Read the model definition and answer for the solid it produces. Units are mm, in the model's axes. Face numbers are marked on the shaded views. A direction names the side the tool comes from. Coordinates: 2 decimals unless noted, no trailing zeros. Loops run counter-clockwise (first coordinate to the right, second up) from the corner with the lowest first, then second, coordinate; pieces in that order, holes last. Notation, with made-up numbers: (-40, -24.75) -> (-9, -24.75) arc R20 cw to (-9, -18.75) -> close; hole circle Ø3 at (-19.5, 78). An arc over 180 degrees is marked (long way). Answer as a JSON object with one key per item and string values. Group by question number.
1) Section A-A, the plane y = 0 is taken. Give the vertices of the cut face in (x, z), plus the area to 3 significant figures.
2) Section D-D, the plane x = -38.5 is taken. Give the vertices of the cut face in (y, z).
3) Flat-ended cylindrical pins translate along their axes: P1, Ø4, axis at x = -9.5, z = 15.5, coming from the +Y side; P2, Ø4, axis at x = 33.64, y = 46.31, coming from the +Z side; P3, Ø6.5, axis at x = 54.44, y = -17.69, coming from the +Z side; P4, Ø2, axis at y = -8.5, z = 6.5, coming from the +X side. Find the tip coordinate at first contact, or state that the pin passes through.
4) Determine the mould class of the marked faces 4, 5 and 6 for opening direction X: released by +X, released by -X, zero draft, split by the parting line, or undercut.
5) Consider probe 1 along Y at (x, z) = (-35.5, 4.75); probe 2 along Y at (x, z) = (-0.5, 4.75); probe 3 along Z at (x, y) = (-25, 16). Determine where each line is inside the solid, lowest interval first. Write a range as [from, to].
6) Section B-B, the plane x = 0 is taken. Count the separate pieces of the cut face and the enclosed holes in it, plus the area to 4 significant figures.
7) Section C-C, the plane z = 9.25 is taken. Give the vertices of the cut face in (x, y), plus the area to 3 significant figures.
8) Which of the six approach directions +Z, -Z, +X, -X, +Y, -Y give full straight-line access (tool end or side, diameter ignored) to the marked faces 1, 2 and 3?
from build123d import *

# Parameters (mm, degrees)
SKETCH1_R           = 63.5
BOSS_EXTRUDE1_DEPTH = 5
SKETCH2_R           = 51
BOSS_EXTRUDE2_DEPTH = 13
SKETCH3_R           = 36
CUT_EXTRUDE1_DEPTH  = 19
CUT_EXTRUDE3_START  = -2.5
SKETCH4_R           = 37.5
SKETCH4_R_2         = 36
CUT_EXTRUDE3_DEPTH  = 2
SKETCH6_R           = 36
SKETCH6_R_2         = 34
BOSS_EXTRUDE6_DEPTH = 2
SKETCH9_R           = 2.5
CUT_EXTRUDE9_DEPTH  = 6
SKETCH10_R          = 2.5
CUT_EXTRUDE10_DEPTH = 19
CUT_EXTRUDE11_DEPTH = 19
FILLET1_R           = 3
FILLET2_R           = 3
FILLET3_R           = 3


with BuildPart() as part:
    # Sketch1 → Boss-Extrude1 (new body)
    with BuildSketch(Plane.XY):
        Circle(SKETCH1_R)
    extrude(amount=BOSS_EXTRUDE1_DEPTH)

    # Sketch2 → Boss-Extrude2 (add)
    with BuildSketch(Plane.XY.offset(5)):
        Circle(SKETCH2_R)
    extrude(amount=BOSS_EXTRUDE2_DEPTH)

    # Sketch3 → Cut-Extrude1 (cut, through all)
    with BuildSketch(Plane.XY.offset(18)):
        with Locations((7.5, 0)):
            Circle(SKETCH3_R)
    extrude(amount=-CUT_EXTRUDE1_DEPTH, mode=Mode.SUBTRACT)

    # Sketch4 → Cut-Extrude3 (cut)
    with BuildSketch(Plane.XY.offset(18).offset(CUT_EXTRUDE3_START)):
        with Locations((7.5, 0)):
            Circle(SKETCH4_R)
        with Locations((7.5, 0)):
            Circle(SKETCH4_R_2, mode=Mode.SUBTRACT)
    extrude(amount=-CUT_EXTRUDE3_DEPTH, mode=Mode.SUBTRACT)

    # Sketch6 → Boss-Extrude6 (add)
    with BuildSketch(Plane(origin=(0, 0, 0), x_dir=(-1, 0, 0), z_dir=(0, 0, -1))):
        with Locations((-7.5, 0)):
            Circle(SKETCH6_R)
        with Locations((-7.5, 0)):
            Circle(SKETCH6_R_2, mode=Mode.SUBTRACT)
    extrude(amount=-BOSS_EXTRUDE6_DEPTH)

    # Sketch9 → Cut-Extrude9 (cut, through all)
    with BuildSketch(Plane.XY.offset(5)):
        with Locations((0, 57.24)):
            Circle(SKETCH9_R)
        with Locations((11.900865182, 55.989168666)):
            Circle(SKETCH9_R)
        with Locations((23.28160545, 52.291341995)):
            Circle(SKETCH9_R)
        with Locations((33.644827841, 46.308132758)):
            Circle(SKETCH9_R)
        with Locations((42.53760981, 38.301035908)):
            Circle(SKETCH9_R)
        with Locations((49.571294113, 28.62)):
            Circle(SKETCH9_R)
        with Locations((54.438474993, 17.688132758)):
            Circle(SKETCH9_R)
        with Locations((56.926433291, 5.983209237)):
            Circle(SKETCH9_R)
        with Locations((56.926433291, -5.983209237)):
            Circle(SKETCH9_R)
        with Locations((54.438474993, -17.688132758)):
            Circle(SKETCH9_R)
        with Locations((49.571294113, -28.62)):
            Circle(SKETCH9_R)
        with Locations((42.53760981, -38.301035908)):
            Circle(SKETCH9_R)
        with Locations((33.644827841, -46.308132758)):
            Circle(SKETCH9_R)
        with Locations((23.28160545, -52.291341995)):
            Circle(SKETCH9_R)
        with Locations((11.900865182, -55.989168666)):
            Circle(SKETCH9_R)
        with Locations((0, -57.24)):
            Circle(SKETCH9_R)
        with Locations((-11.900865182, -55.989168666)):
            Circle(SKETCH9_R)
        with Locations((-23.28160545, -52.291341995)):
            Circle(SKETCH9_R)
        with Locations((-33.644827841, -46.308132758)):
            Circle(SKETCH9_R)
        with Locations((-42.53760981, -38.301035908)):
            Circle(SKETCH9_R)
        with Locations((-49.571294113, -28.62)):
            Circle(SKETCH9_R)
        with Locations((-54.438474993, -17.688132758)):
            Circle(SKETCH9_R)
        with Locations((-56.926433291, -5.983209237)):
            Circle(SKETCH9_R)
        with Locations((-56.926433291, 5.983209237)):
            Circle(SKETCH9_R)
        with Locations((-54.438474993, 17.688132758)):
            Circle(SKETCH9_R)
        with Locations((-49.571294113, 28.62)):
            Circle(SKETCH9_R)
        with Locations((-42.53760981, 38.301035908)):
            Circle(SKETCH9_R)
        with Locations((-33.644827841, 46.308132758)):
            Circle(SKETCH9_R)
        with Locations((-23.28160545, 52.291341995)):
            Circle(SKETCH9_R)
        with Locations((-11.900865182, 55.989168666)):
            Circle(SKETCH9_R)
    extrude(amount=-CUT_EXTRUDE9_DEPTH, mode=Mode.SUBTRACT)

    # Sketch10 → Cut-Extrude10 (cut, through all)
    with BuildSketch(Plane.XY.offset(18)):
        with Locations((-38.5, 0)):
            Circle(SKETCH10_R)
    extrude(amount=-CUT_EXTRUDE10_DEPTH, mode=Mode.SUBTRACT)

    # Sketch11 → Cut-Extrude11 (cut, through all)
    with BuildSketch(Plane.XY.offset(18)):
        with BuildLine():
            ThreePointArc((-15.443057454, 32.766081772), (-25.855432883, 22.077479412), (-31.625904029, 8.316467633))
            Line((-31.625904029, 8.316467633), (-44.644725504, 11.083703562))
            ThreePointArc((-44.644725504, 11.083703562), (-36.095276344, 28.515452402), (-21.115563753, 40.867260336))
            Line((-21.115563753, 40.867260336), (-15.443057454, 32.766081772))
        make_face()
    cut_extrude11 = extrude(amount=-CUT_EXTRUDE11_DEPTH, mode=Mode.SUBTRACT)

    # Mirror1: Cut-Extrude11 across plane
    add(cut_extrude11.mirror(Plane.ZX), mode=Mode.SUBTRACT)

    # Fillet1
    fillet1_edges = [part.edges().sort_by_distance(p)[0] for p in [
        (-44.644725504, 11.083703562, 9),
    ]]
    fillet(fillet1_edges, radius=FILLET1_R)

    # Fillet2
    fillet2_edges = [part.edges().sort_by_distance(p)[0] for p in [
        (-15.443057454, 32.766081772, 9),
        (-31.625904029, 8.316467633, 9),
        (-21.115563753, 40.867260336, 9),
    ]]
    fillet(fillet2_edges, radius=FILLET2_R)

    # Fillet3
    fillet3_edges = [part.edges().sort_by_distance(p)[0] for p in [
        (-31.625904029, -8.316467633, 9),
        (-15.443057454, -32.766081772, 9),
        (-21.115563753, -40.867260336, 9),
        (-44.644725504, -11.083703562, 9),
    ]]
    fillet(fillet3_edges, radius=FILLET3_R)


solid = part.part
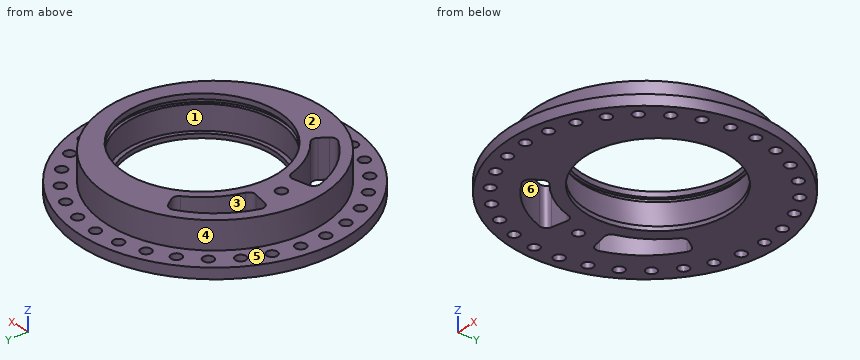
Determined:
{
 "1": {"outline": "(-63.5, 0) -> (-41, 0) -> (-41, 18) -> (-51, 18) -> (-51, 5) -> (-63.5, 5) -> close; (-36, 0) -> (-26.5, 0) -> (-26.5, 2) -> (-28.5, 2) -> (-28.5, 13.5) -> (-30, 13.5) -> (-30, 15.5) -> (-28.5, 15.5) -> (-28.5, 18) -> (-36, 18) -> close; (41.5, 0) -> (63.5, 0) -> (63.5, 5) -> (51, 5) -> (51, 18) -> (43.5, 18) -> (43.5, 15.5) -> (45, 15.5) -> (45, 13.5) -> (43.5, 13.5) -> (43.5, 2) -> (41.5, 2) -> close", "area": "577 mm²"},
 "2": {"outline": "(-50.5, 0) -> (-25.17, 0) -> (-25.17, 18) -> (-33.45, 18) -> (-33.45, 5) -> (-50.5, 5) -> close; (-9.78, 0) -> (-2.5, 0) -> (-2.5, 18) -> (-9.78, 18) -> close; (2.5, 0) -> (9.78, 0) -> (9.78, 18) -> (2.5, 18) -> close; (25.17, 0) -> (50.5, 0) -> (50.5, 5) -> (33.45, 5) -> (33.45, 18) -> (25.17, 18) -> close"},
 "3": {"P1": "y = 50.45", "P2": "through", "P3": "z = 5", "P4": "x = 50.45"},
 "4": {"face 4": "split by the parting line", "face 5": "zero draft", "face 6": "undercut"},
 "5": {"probe 1": "[-52.65, -47.98], [-44.63, -29.25], [-9.14, 9.14], [29.25, 44.63], [47.98, 52.65]", "probe 2": "[-63.5, -59.69], [-54.79, -35.1], [35.1, 54.79], [59.69, 63.5]", "probe 3": "[0, 13.5], [15.5, 18]"},
 "6": {"separate pieces": "4", "enclosed holes": "0", "area": "645.5 mm²"},
 "7": {"outline": "circle Ø102 at (0, 0); hole (-43.73, -14.28) arc R46 ccw to (-23.56, -39.51) arc R3 ccw to (-19.57, -38.65) -> (-17.1, -35.14) arc R3 ccw to (-17.67, -31.09) arc R40 cw to (-30.95, -11.03) arc R3 ccw to (-34.46, -8.92) -> (-41.5, -10.42) arc R3 ccw to start; hole (-43.73, 14.28) arc R3 ccw to (-41.5, 10.42) -> (-34.46, 8.92) arc R3 ccw to (-30.95, 11.03) arc R40 cw to (-17.67, 31.09) arc R3 ccw to (-17.1, 35.14) -> (-19.57, 38.65) arc R3 ccw to (-23.56, 39.51) arc R46 ccw to start; hole circle Ø5 at (-38.5, 0); hole circle Ø72 at (7.5, 0)", "area": "3,270 mm²"},
 "8": {"face 1": "+Z", "face 2": "+Z, +X, -X, +Y, -Y", "face 3": "+Z, -Z"}
}
